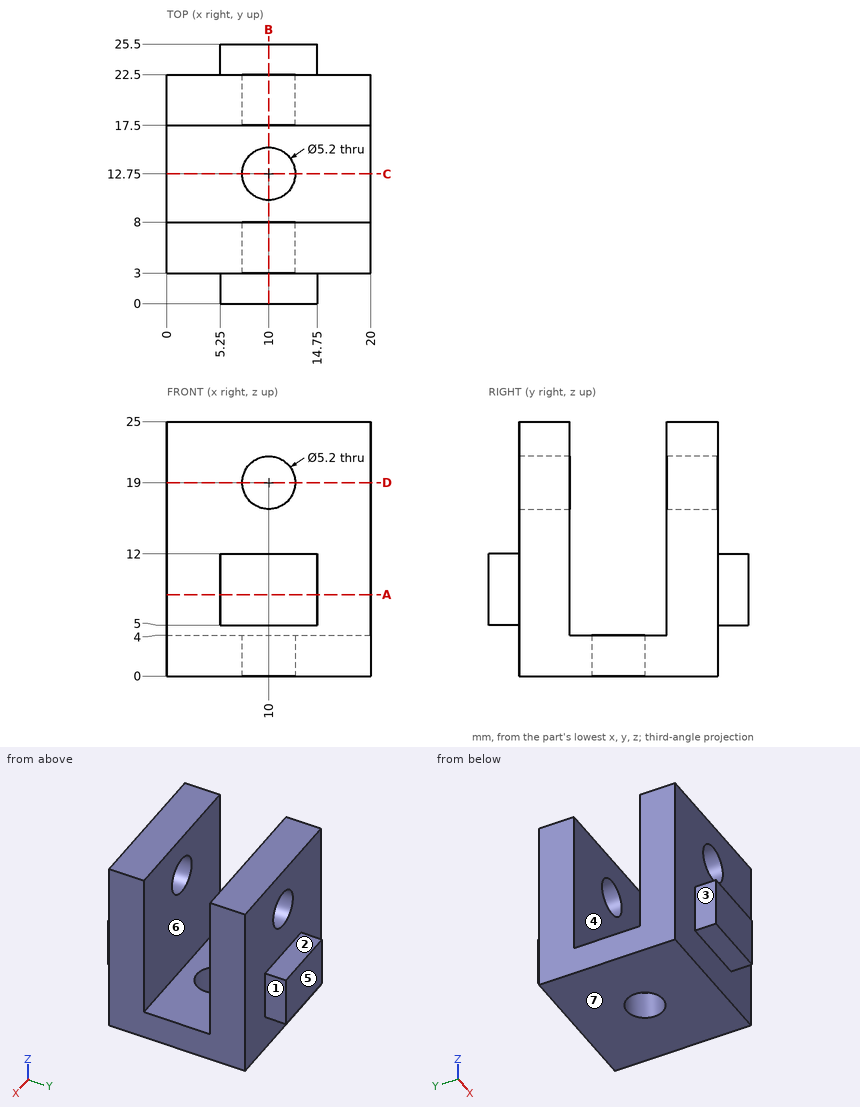
Geometry check sheet. Reference: drawing and pictorial views, mm from the part's lowest x, y, z. A direction names the side the tool comes from. Coordinates: 2 decimals unless noted, no trailing zeros. Write each loop counter-clockwise with the first axis right and the second up, starting at its lowest first coordinate (ties: lowest second). Pieces come first, ordered by that corner, then holes. Notation, with made-up numbers: (20, -11) -> (31, -11) arc R15 ccw to (31, 15) -> close; hole circle Ø10 at (68, 71.25). An arc over 180 degrees is marked (long way). Use a Markdown table: item, result.
1. Sectioned sample at D-D (z = 19). Enter the section's corners in (x, y), plus the area to 3 significant figures.
Reported:
| item | result |
|---|---|
| outline | (0, 3) -> (7.4, 3) -> (7.4, 8) -> (0, 8) -> close; (0, 17.5) -> (7.4, 17.5) -> (7.4, 22.5) -> (0, 22.5) -> close; (12.6, 3) -> (20, 3) -> (20, 8) -> (12.6, 8) -> close; (12.6, 17.5) -> (20, 17.5) -> (20, 22.5) -> (12.6, 22.5) -> close |
| area | 148 mm2 |
2. Go/stop test with flat-tipped pins: pin 1 Ø1.5 at (y, z) = (21, 2.5) entering from -X; pin 2 Ø10 at (x, z) = (12.5, 19) entering from +Y; pin 3 Ø0.9 at (x, y) = (10.5, 1.5) entering from +Z; pin 4 Ø0.9 at (x, y) = (10, 24) entering from -Z. Record where each tip stops, or that it passes through.
Reported:
| item | result |
|---|---|
| pin 1 | stops at x = 0 |
| pin 2 | stops at y = 22.5 |
| pin 3 | stops at z = 12 |
| pin 4 | stops at z = 5 |
3. Scan lines: line 1 along Y through (x, z) = (1.5, 11.25); line 2 along Y through (x, z) = (14, 5.25); line 3 along X through (y, z) = (21.4, 19). Record each from-to range of solid material in increasing order.
Reported:
| item | result |
|---|---|
| line 1 | y = 3 to 8, 17.5 to 22.5 |
| line 2 | y = 0 to 8, 17.5 to 25.5 |
| line 3 | x = 0 to 7.4, 12.6 to 20 |
4. Release check for a two-part mould opening along Y. For the marked faces 5, 6 and 7 record: pulls with the +Y half, pulls with the -Y half, needs draft (parallel to the pull), parting line crosses it, or undercut.
Reported:
| item | result |
|---|---|
| face 5 | pulls with the +Y half |
| face 6 | undercut |
| face 7 | needs draft |
5. Sectioned sample at C-C (y = 12.75). Enter the section's corners in (x, z).
Reported:
| item | result |
|---|---|
| outline | (0, 0) -> (7.4, 0) -> (7.4, 4) -> (0, 4) -> close; (12.6, 0) -> (20, 0) -> (20, 4) -> (12.6, 4) -> close |
6. Tool access check on the marked faces 1, 2, 3 and 4. Record the directions out of +Z, -Z, +X, -X, +Y, -Y that give a thin tool (end or side, any length) a straight path to the whole face; none if there is none.
Reported:
| item | result |
|---|---|
| face 1 | +Z, -Z, +X, +Y |
| face 2 | +Z, +X, -X, +Y |
| face 3 | +Z, -Z, -X, -Y |
| face 4 | +Z, +X, -X |
7. Sectioned sample at B-B (x = 10). Enter the section's corners in (y, z).
Reported:
| item | result |
|---|---|
| outline | (0, 5) -> (3, 5) -> (3, 0) -> (10.15, 0) -> (10.15, 4) -> (8, 4) -> (8, 16.4) -> (3, 16.4) -> (3, 12) -> (0, 12) -> close; (3, 21.6) -> (8, 21.6) -> (8, 25) -> (3, 25) -> close; (15.35, 0) -> (22.5, 0) -> (22.5, 5) -> (25.5, 5) -> (25.5, 12) -> (22.5, 12) -> (22.5, 16.4) -> (17.5, 16.4) -> (17.5, 4) -> (15.35, 4) -> close; (17.5, 21.6) -> (22.5, 21.6) -> (22.5, 25) -> (17.5, 25) -> close |
8. Sectioned sample at A-A (z = 8). Enter the section's corners in (x, y), plus the area to 3 significant figures.
Reported:
| item | result |
|---|---|
| outline | (0, 3) -> (5.25, 3) -> (5.25, 0) -> (14.75, 0) -> (14.75, 3) -> (20, 3) -> (20, 8) -> (0, 8) -> close; (0, 17.5) -> (20, 17.5) -> (20, 22.5) -> (14.75, 22.5) -> (14.75, 25.5) -> (5.25, 25.5) -> (5.25, 22.5) -> (0, 22.5) -> close |
| area | 257 mm2 |
